The model under review builds one solid part; all positions refer to its coordinate system, in mm. A direction names the side the tool comes from. Coordinates: 2 decimals unless noted, no trailing zeros. Order: outer loops, then holes, each group sorted by start corner. A loop starts at its lowest first (then second) coordinate and runs counter-clockwise, first axis right, second up. Notation, with made-up numbers: (-5.75, 70.5) -> (37.25, 70.5) arc R15 cw to (37.25, 82.5) -> close; hole circle Ø2 at (-3, 33.5). An arc over 180 degrees is marked (long way). Answer as CSV lines item,"result". Start each with the question number.
from build123d import *

# Parameters (mm, degrees)
SKETCH1_W           = 60
SKETCH1_H           = 45
BOSS_EXTRUDE1_DEPTH = 4
SKETCH2_W           = 10
SKETCH2_H           = 5
BOSS_EXTRUDE3_DEPTH = 62
SKETCH3_R           = 18
BOSS_EXTRUDE4_DEPTH = 61
SKETCH4_R           = 6
CUT_EXTRUDE1_DEPTH  = 4
SCALE1_SCALE        = 0.15


with BuildPart() as part:
    # Sketch1 → Boss-Extrude1 (new body)
    with BuildSketch(Plane.XY):
        with Locations((0.693972483, 0.258252113)):
            Rectangle(SKETCH1_W, SKETCH1_H)
    extrude(amount=BOSS_EXTRUDE1_DEPTH)

    # Sketch2 → Boss-Extrude3 (add)
    with BuildSketch(Plane(origin=(0, 0, 0), x_dir=(-1, 0, 0), z_dir=(0, 0, -1))):
        with Locations((-25.693972483, -19.741747887)):
            Rectangle(SKETCH2_W, SKETCH2_H)
        with Locations((24.306027517, -19.741747887)):
            Rectangle(SKETCH2_W, SKETCH2_H)
    extrude(amount=BOSS_EXTRUDE3_DEPTH)

    # Sketch3 → Boss-Extrude4 (add)
    with BuildSketch(Plane(origin=(0, 0, 0), x_dir=(-1, 0, 0), z_dir=(0, 0, -1))):
        with Locations(Location((-0.693972483, -4.241747887, 0), (0, 0, 270))):
            Circle(SKETCH3_R)
    extrude(amount=BOSS_EXTRUDE4_DEPTH)

    # Sketch4 → Cut-Extrude1 (cut)
    with BuildSketch(Plane.XY.offset(4)):
        with Locations((0.693972483, -10.241747887)):
            Circle(SKETCH4_R)
    extrude(amount=-CUT_EXTRUDE1_DEPTH, mode=Mode.SUBTRACT)


with BuildPart() as part_1:
    # Scale1: scaled about (0.693972483, -4.811264364, -26.262899062)
    add(part.part.scale(SCALE1_SCALE).moved(Location((0.589876611, -4.089574709, -22.323464203))))


solid = part_1.part
1) Insertion check: pin 1 Ø1 at (x, z) = (0.5, -23.5) entering from +Y; pin 2 Ø2 at (x, z) = (4, -27.5) entering from +Y; pin 3 Ø2.5 at (x, y) = (1, -5) entering from -Z. Each pin has a flat end and moves straight along its axis. Give the tip position at first contact, or say it passes through.
2) Consider section D-D (x = 2). Give the boundary of the cut face in (y, z).
3) Consider section B-B (x = -2.75). Give the boundary of the cut face in (y, z).
4) Wall thickness on L1, parallel to X at y = -7, z = -29.5; L2, parallel to Z at x = 0, y = -4.75; L3, parallel to Y at x = 4.25, z = -22.5: over which ranges is each line inside the solid? List them lowest first. Write a range as [from, to].
5) Consider section C-C (y = -6). Give the boundary of the cut face in (x, z).
6) Mouldability with a two-part tool opening along X and no side actions: class faces 6 (the face through (-3.806, -7, -25)), 7 (the face through (-0.12, -7.3, -26.83)), 8 (the face through (5.194, -7, -25)) as released by +X, released by -X, zero draft, split by the parting line, or undercut.
7) Consider section A-A (z = -26). Give the boundary of the cut face in (x, y), plus the area to 3 significant figures.
8) Tool access review of faces 1 (the face through (1, -4, -21.723)), 2 (the face through (-3, -6.676, -27)), 3 (the face through (4, -7.426, -26)), 4 (the face through (0.499, -6.504, -22.019)), 5 (the face through (4, -6.676, -27)): name each direction out of +Z, -Z, +X, -X, +Y, -Y from which nothing blocks a thin tool from reaching the whole face with its end or side.
Result:
1,pin 1,"y = -2.03"
1,pin 2,"y = -3.32"
1,pin 3,"z = -31.47"
2,outline,"(-7.43, -22.32) -> (-7.09, -22.32) -> (-7.09, -31.47) -> (-2.36, -31.47) -> (-2.36, -22.32) -> (-0.68, -22.32) -> (-0.68, -21.72) -> (-7.43, -21.72) -> close"
3,outline,"(-7.43, -31.62) -> (-6.68, -31.62) -> (-6.68, -22.32) -> (-0.68, -22.32) -> (-0.68, -21.72) -> (-7.43, -21.72) -> close"
4,L1,"[-3.81, -2.31], [-0.76, 2.15], [3.69, 5.19]"
4,L2,"[-31.47, -21.72]"
4,L3,"[-7.43, -6.68]"
5,outline,"(-3.81, -22.32) -> (-1.69, -22.32) -> (-1.69, -31.47) -> (3.07, -31.47) -> (3.07, -22.32) -> (5.19, -22.32) -> (5.19, -21.72) -> (1.51, -21.72) -> (1.51, -22.32) -> (-0.12, -22.32) -> (-0.12, -21.72) -> (-3.81, -21.72) -> close"
6,face 6,"released by -X"
6,face 7,"undercut"
6,face 8,"released by +X"
7,outline,"(-3.81, -7.43) -> (-2.31, -7.43) -> (-2.31, -6.68) -> (-3.81, -6.68) -> close; circle Ø5.4 at (0.69, -4.73); (3.69, -7.43) -> (5.19, -7.43) -> (5.19, -6.68) -> (3.69, -6.68) -> close"
7,area,"25.2 mm2"
8,face 1,"+Z, +X, -X, +Y, -Y"
8,face 2,"-Z, -X, +Y"
8,face 3,"+Z, -Z, +X, -X, -Y"
8,face 4,"+Z"
8,face 5,"-Z, +X, +Y"
